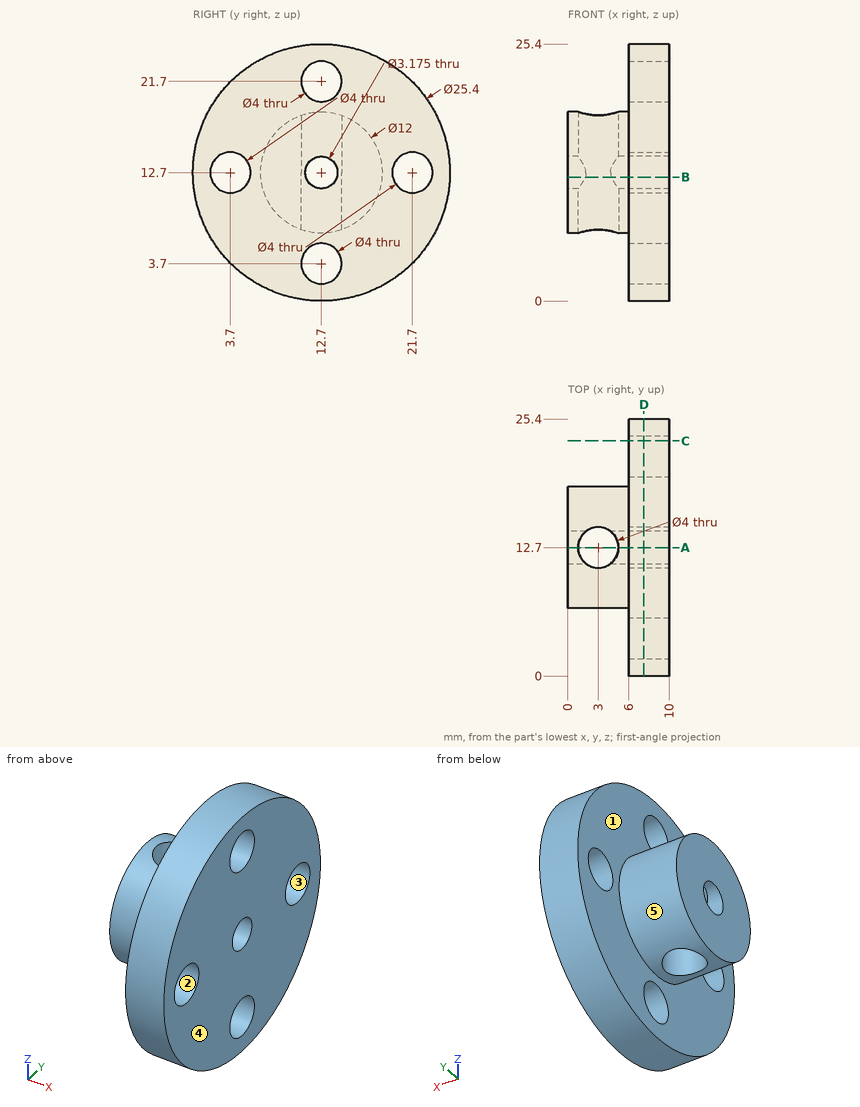
Geometry check sheet. Reference: drawing and pictorial views, mm from the part's lowest x, y, z. A direction names the side the tool comes from. Coordinates: 2 decimals unless noted, no trailing zeros. Loops run counter-clockwise (first coordinate to the right, second up) from the corner with the lowest first, then second, coordinate; pieces in that order, holes last. Notation, with made-up numbers: (36.25, -30.5) -> (88.25, -30.5) arc R24 ccw to (88.25, 1.5) -> close; hole circle Ø2 at (-28.5, 46.25). An arc over 180 degrees is marked (long way). Put each result on its own line as item: value.
1) Cross-section at B-B on z = 12.25. Record the boundary of the cut face in (x, y), plus the area to 3 significant figures.
Result set:
outline: (0, 6.72) -> (6, 6.72) -> (6, 5.65) -> (10, 5.65) -> (10, 11.18) -> (4.3, 11.18) arc R2 cw to (1.7, 11.18) -> (0, 11.18) -> close; (0, 14.22) -> (1.7, 14.22) arc R2 cw to (4.3, 14.22) -> (10, 14.22) -> (10, 19.75) -> (6, 19.75) -> (6, 18.68) -> (0, 18.68) -> close; (6, 0.01) -> (10, 0.01) -> (10, 1.75) -> (6, 1.75) -> close; (6, 23.65) -> (10, 23.65) -> (10, 25.39) -> (6, 25.39) -> close
area: 110 mm^2
2) Thickness scan on line 1 (X direction, y = 12.7, z = 17.75); line 2 (Y direction, x = 0.4, z = 12.7); line 3 (X direction, y = 18.5, z = 19). Record the ranges inside material, lowest first.
Result set:
line 1: x = 0 to 1, 5 to 10
line 2: y = 6.7 to 11.11, 14.29 to 18.7
line 3: x = 6 to 10
3) Cross-section at D-D on x = 7.5. Record the boundary of the cut face in (y, z) (1 decimal).
Result set:
outline: circle Ø25.4 at (12.7, 12.7); hole circle Ø4 at (3.7, 12.7); hole circle Ø4 at (12.7, 3.7); hole circle Ø4 at (12.7, 21.7); hole circle Ø3.2 at (12.7, 12.7); hole circle Ø4 at (21.7, 12.7)
4) Release check for a two-part mould opening along Z. For the marked faces 3, 4 and 5 record: released by +Z, released by -Z, zero draft, split by the parting line, or undercut.
Result set:
face 3: undercut
face 4: zero draft
face 5: split by the parting line
5) Tool access check on the marked faces 1 and 2. Record the directions out of +Z, -Z, +X, -X, +Y, -Y that give a thin tool (end or side, any length) a straight path to the whole face; none if there is none.
Result set:
face 1: -X
face 2: +X, -X
6) Gauge pin test, flat ends, axial feed: pin 1 Ø5 at (x, z) = (8.5, 8.5) entering from -Y; pin 2 Ø5 at (x, y) = (3, 12.7) entering from +Z; pin 3 Ø5 at (y, z) = (12.7, 3.7) entering from -X; pin 4 Ø1.9 at (y, z) = (12.7, 12.7) entering from -X. Record the tip position at first contact, or that the pin passes through.
Result set:
pin 1: stops at y = 0.11
pin 2: stops at z = 18.7
pin 3: stops at x = 6
pin 4: passes through
7) Cross-section at A-A on y = 12.7. Record the boundary of the cut face in (x, z).
Result set:
outline: (0, 6.7) -> (1, 6.7) -> (1, 11.11) -> (0, 11.11) -> close; (0, 14.29) -> (1, 14.29) -> (1, 18.7) -> (0, 18.7) -> close; (5, 6.7) -> (6, 6.7) -> (6, 5.7) -> (10, 5.7) -> (10, 11.11) -> (5, 11.11) -> close; (5, 14.29) -> (10, 14.29) -> (10, 19.7) -> (6, 19.7) -> (6, 18.7) -> (5, 18.7) -> close; (6, 0) -> (10, 0) -> (10, 1.7) -> (6, 1.7) -> close; (6, 23.7) -> (10, 23.7) -> (10, 25.4) -> (6, 25.4) -> close
8) Cross-section at C-C on y = 23.25. Record the boundary of the cut face in (x, z), plus the area to 4 significant figures.
Result set:
outline: (6, 5.63) -> (10, 5.63) -> (10, 11.44) -> (6, 11.44) -> close; (6, 13.96) -> (10, 13.96) -> (10, 19.77) -> (6, 19.77) -> close
area: 46.45 mm^2
